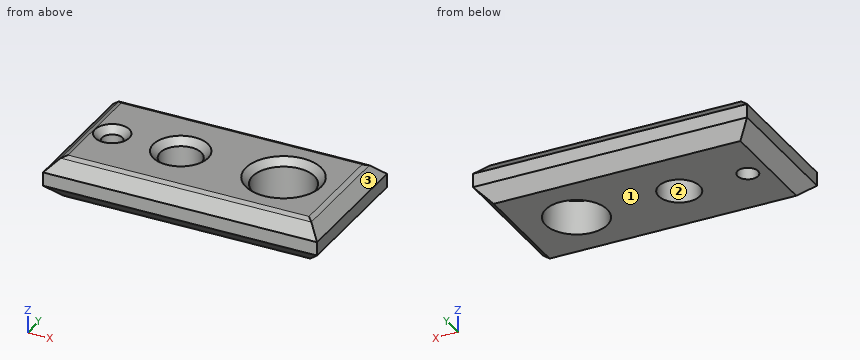
```python
from build123d import *

# Parameters (mm, degrees)
F0_W        = 200
F0_H        = 100
F1_DEPTH    = 15
F2_C1_SIZE  = 10
F2_C2_SIZE  = 10
F2_C3_SIZE  = 10
F2_C4_SIZE  = 10
F2_C5_SIZE  = 10
F2_C6_SIZE  = 10
F2_C7_SIZE  = 10
F2_C8_SIZE  = 10
F3_R        = 15
F3_R_2      = 7.5
F3_R_3      = 22.5
F4_DEPTH    = 30.001
F5_T1_DEPTH = 91.2857086021
F5_T3_DEPTH = 191.2857086021


# Not quite as in the source:
# - a fillet or chamfer that OpenCascade refuses, or shapes differently, is made with other operations: its cross-section is extruded or revolved along the edge and cut away or added


with BuildPart() as f1:
    # F0 (on Top) → F1 (new body, symmetric)
    with BuildSketch(Plane.XY):
        Rectangle(F0_W, F0_H)
    extrude(amount=F1_DEPTH, both=True)

    # F2: chamfer of 10 on 8 edges, made by hand

    # F2_c1
    f2_c1_edges = [f1.edges().sort_by_distance(p)[0] for p in [
        (100, 0, -15),
    ]]
    chamfer(f2_c1_edges, length=F2_C1_SIZE)

    # F2_c2
    f2_c2_edges = [f1.edges().sort_by_distance(p)[0] for p in [
        (100, 0, 15),
    ]]
    chamfer(f2_c2_edges, length=F2_C2_SIZE)

    # F2_c3
    f2_c3_edges = [f1.edges().sort_by_distance(p)[0] for p in [
        (-5, -50, -15),
    ]]
    chamfer(f2_c3_edges, length=F2_C3_SIZE)

    # F2_c4
    f2_c4_edges = [f1.edges().sort_by_distance(p)[0] for p in [
        (-5, -50, 15),
    ]]
    chamfer(f2_c4_edges, length=F2_C4_SIZE)

    # F2_c5
    f2_c5_edges = [f1.edges().sort_by_distance(p)[0] for p in [
        (-100, 5, -15),
    ]]
    chamfer(f2_c5_edges, length=F2_C5_SIZE)

    # F2_c6
    f2_c6_edges = [f1.edges().sort_by_distance(p)[0] for p in [
        (-100, 5, 15),
    ]]
    chamfer(f2_c6_edges, length=F2_C6_SIZE)

    # F2_c7
    f2_c7_edges = [f1.edges().sort_by_distance(p)[0] for p in [
        (0, 50, 15),
    ]]
    chamfer(f2_c7_edges, length=F2_C7_SIZE)

    # F2_c8
    f2_c8_edges = [f1.edges().sort_by_distance(p)[0] for p in [
        (0, 50, -15),
    ]]
    chamfer(f2_c8_edges, length=F2_C8_SIZE)

    # F3 (on face) → F4 (cut, through all)
    with BuildSketch(Plane.XY.offset(15)):
        with Locations((-25, 0)):
            Circle(F3_R)
        with Locations((-75, 0)):
            Circle(F3_R_2)
        with Locations((50, 0)):
            Circle(F3_R_3)
    extrude(amount=-F4_DEPTH, mode=Mode.SUBTRACT)

    # F5: chamfer of 5 on 7 edges, made by hand

    # F5_s2 → F5_t1 (cut)
    with BuildSketch(Plane.XZ.offset(-45.6428543011)):
        Polygon((-91.4644660941, 13.5355339059), (-87.9289321881, 15), (-90, 15), align=None)
        Polygon((91.4644660941, 13.5355339059), (87.9289321881, 15), (90, 15), align=None)
    extrude(amount=F5_T1_DEPTH, mode=Mode.SUBTRACT)

    # F5_s4 → F5_t3 (cut)
    with BuildSketch(Plane.YZ.offset(-95.6428543011)):
        Polygon((41.4644660941, 13.5355339059), (37.9289321881, 15), (40, 15), align=None)
        Polygon((-37.9289321881, 15), (-41.4644660941, 13.5355339059), (-40, 15), align=None)
    extrude(amount=F5_T3_DEPTH, mode=Mode.SUBTRACT)

    # F5_s5 → F5_t6 (revolve, cut)
    with BuildSketch(Plane.XZ):
        Polygon((77.5, 15), (72.5, 10), (72.5, 15), align=None)
    revolve(axis=Axis((50, 0, 15), (0, 0, 1)), mode=Mode.SUBTRACT)

    # F5_s7 → F5_t8 (revolve, cut)
    with BuildSketch(Plane.XZ):
        Polygon((-5, 15), (-10, 10), (-10, 15), align=None)
    revolve(axis=Axis((-25, 0, 15), (0, 0, 1)), mode=Mode.SUBTRACT)

    # F5_s9 → F5_t10 (revolve, cut)
    with BuildSketch(Plane.XZ):
        Polygon((-62.5, 15), (-67.5, 10), (-67.5, 15), align=None)
    revolve(axis=Axis((-75, 0, 15), (0, 0, 1)), mode=Mode.SUBTRACT)


solid = f1.part
```
Here's how the part is built. I have some questions about the finished solid (model axes, mm). Face numbers are marked on the shaded views. Coordinates: 2 decimals unless noted, no trailing zeros. Write each loop counter-clockwise with the first axis right and the second up, starting at its lowest first coordinate (ties: lowest second). Pieces come first, ordered by that corner, then holes. Notation, with made-up numbers: (64, -30.5) -> (74, -30.5) arc R5 ccw to (74, -22.5) -> close; hole circle Ø8 at (23, 22.25). An arc over 180 degrees is marked (long way). Use a Markdown table: item, result. Add a question column.
(1) We'd pull the mould along X, two halves only. Please class the marked faces 1, 2 and 3: +X half, -X half, draft (parallel to the pull), parting line (faces both ways), or undercut.
(2) I'm going to push flat-ended pins straight in: P1, Ø1, axis at y = -23.5, z = -7, coming from the +X side; P2, Ø12, axis at x = -75, y = 0, coming from the +Z side; P3, Ø2, axis at y = 20.5, z = -8.5, coming from the -X side. Where does each tip first touch, or does it pass through?
(3) If we section it at A-A, the plane x = 50: Write out the boundary of the cut face in (y, z), and give its area (3 significant figures).
(4) If we section it at B-B, the plane y = 0: Write out the boundary of the cut face in (x, z), and give its area (3 significant figures).
(5) If we section it at C-C, the plane z = 7.5: Write out the boundary of the cut face in (x, y), and give its area (3 significant figures).
(6) Please list where these lines run through material, in increasing order: line 1 (Y direction, x = 50, z = -1); line 2 (Y direction, x = -75, z = 3); line 3 (X direction, y = -13, z = 2).
(7) If we section it at D-D, the plane y = 32: Write out the boundary of the cut face in (x, z), and give its area (3 significant figures).
Outcome:
| question | item | result |
|---|---|---|
| 1 | face 1 | draft |
| 1 | face 2 | undercut |
| 1 | face 3 | +X half |
| 2 | P1 | stops at x = 98.5 |
| 2 | P2 | passes through |
| 2 | P3 | stops at x = -97.5 |
| 3 | outline | (-50, -5) -> (-40, -15) -> (-22.5, -15) -> (-22.5, 10) -> (-27.5, 15) -> (-37.93, 15) -> (-41.46, 13.54) -> (-50, 5) -> close; (22.5, -15) -> (40, -15) -> (50, -5) -> (50, 5) -> (41.46, 13.54) -> (37.93, 15) -> (27.5, 15) -> (22.5, 10) -> close |
| 3 | area | 1,420 mm^2 |
| 4 | outline | (-100, -5) -> (-90, -15) -> (-82.5, -15) -> (-82.5, 10) -> (-87.5, 15) -> (-87.93, 15) -> (-91.46, 13.54) -> (-100, 5) -> close; (-67.5, -15) -> (-40, -15) -> (-40, 10) -> (-45, 15) -> (-62.5, 15) -> (-67.5, 10) -> close; (-10, -15) -> (27.5, -15) -> (27.5, 10) -> (22.5, 15) -> (-5, 15) -> (-10, 10) -> close; (72.5, -15) -> (90, -15) -> (100, -5) -> (100, 5) -> (91.46, 13.54) -> (87.93, 15) -> (77.5, 15) -> (72.5, 10) -> close |
| 4 | area | 3,020 mm^2 |
| 5 | outline | (-97.5, -47.5) -> (97.5, -47.5) -> (97.5, 47.5) -> (-97.5, 47.5) -> close; hole circle Ø15 at (-75, 0); hole circle Ø30 at (-25, 0); hole circle Ø45 at (50, 0) |
| 5 | area | 16,100 mm^2 |
| 6 | line 1 | y = -50 to -22.5, 22.5 to 50 |
| 6 | line 2 | y = -50 to -7.5, 7.5 to 50 |
| 6 | line 3 | x = -100 to -32.48, -17.52 to 31.64, 68.36 to 100 |
| 7 | outline | (-100, -5) -> (-90, -15) -> (90, -15) -> (100, -5) -> (100, 5) -> (91.46, 13.54) -> (87.93, 15) -> (-87.93, 15) -> (-91.46, 13.54) -> (-100, 5) -> close |
| 7 | area | 5,800 mm^2 |
